from build123d import *

# Parameters (mm, degrees)
BOSS_EXTRUDE1_DEPTH = 50


with BuildPart() as part:
    # Sketch1 → Boss-Extrude1 (new body)
    with BuildSketch(Plane(origin=(0, 0, 0), x_dir=(1, 0, 0), z_dir=(0, 1, 0))):
        Polygon((-434.22123396, 330.511591748), (-490.415824699, -64.194072769), (-472.477870031, -524.138824529), (-270.660991621, -696.876695154), (273.24324441, -696.876695154), (475.06012282, -524.138824529), (492.998077488, -64.194072769), (436.803486749, 330.511591748), (255.52688097, 580.827312496), (1.291126394, 709.058947943), (-252.944628181, 580.827312496), align=None)
        Polygon((327.5, -536.876695154), (212.5, -536.876695154), (212.5, -411.876695154), (97.5, -411.876695154), (-97.5, -411.876695154), (-212.5, -411.876695154), (-212.5, -536.876695154), (-327.5, -536.876695154), (-327.5, -216.876695154), (-212.5, -216.876695154), (-212.5, -96.876695154), (-212.5, -81.876695154), (-317.5, -81.876695154), (-317.5, 118.123304846), (-202.5, 118.123304846), (-202.5, -81.876695154), (-202.5, -96.876695154), (-97.5, -96.876695154), (-97.5, -66.876695154), (97.5, -66.876695154), (97.5, -96.876695154), (202.5, -96.876695154), (202.5, -81.876695154), (202.5, 118.123304846), (317.5, 118.123304846), (317.5, -81.876695154), (212.5, -81.876695154), (212.5, -96.876695154), (212.5, -216.876695154), (327.5, -216.876695154), align=None, mode=Mode.SUBTRACT)
    extrude(amount=-BOSS_EXTRUDE1_DEPTH)


solid = part.part
Read the model definition and answer for the solid it produces. Units are mm, in the model's axes. A direction names the side the tool comes from. Round coordinates to 2 decimals unless told otherwise and drop trailing zeros. Order: outer loops, then holes, each group sorted by start corner. A loop starts at its lowest first (then second) coordinate and runs counter-clockwise, first axis right, second up.
1) For faces 1 (the face through (-261, -25, -118.123)), 2 (the face through (-124.05, -24.65, -645.84)), determine the directions among +Z, -Z, +X, -X, +Y, -Y from which every point of the face is accessible in a straight line to the end or side of a thin tool.
2) The part is cut by section D-D on z = -436.5. Write down the section's boundary in (x, y), plus the area to 3 significant figures.
3) Flat-ended cylindrical pins translate along their axes: pin 1 (15 mm diameter, centred on y = -25, z = 497, fed in from -X); pin 2 (8 mm diameter, centred on y = -27, z = -256.5, fed in from +X); pin 3 (24 mm diameter, centred on y = -22.5, z = 89.5, fed in from -X). Find the tip coordinate at first contact, or state that the pin passes through.
4) Straight lines are drawn through the part: L1, parallel to Z at x = -242.5, y = -26; L2, parallel to X at y = -31, z = 28.5; L3, parallel to Z at x = -262, y = -46. For each, find the intervals that lie inside material, in ascending order.
5) The part is cut by section B-B on z = 331. Write down the section's boundary in (x, y).
6) The mould has two halves that part along X. Classify faces 3 (the face through (-269, -25, 536.877)), 4 (the face through (-6, 0, -16)), 5 (the face through (327.5, -25, 375)), 6 (the face through (-461.925, -24.65, -135.922)): released by +X, released by -X, zero draft, split by the parting line, or undercut.
7) The part is cut by section A-A on x = -115. Write down the section's boundary in (y, z).
8) The part is cut by section C-C on z = -242.5. Write down the section's boundary in (x, y).
Resolved:
1. face 1: +Y, -Y
1. face 2: -Z, -X, +Y, -Y
2. outline: (-357.47, -50) - (360.05, -50) - (360.05, 0) - (-357.47, 0) - close
2. area: 35,900 mm2
3. pin 1: stops at x = -473.83
3. pin 2: stops at x = 447.91
3. pin 3: stops at x = -489.9
4. L1: z = -586.1 to -118.12, 81.88 to 216.88, 536.88 to 696.88
4. L2: x = -485.33 to -317.5, -202.5 to 202.5, 317.5 to 487.92
4. L3: z = -568.32 to -118.12, 81.88 to 216.88, 536.88 to 696.88
5. outline: (-480.01, -50) - (-327.5, -50) - (-327.5, 0) - (-480.01, 0) - close; (327.5, -50) - (482.59, -50) - (482.59, 0) - (327.5, 0) - close
6. face 3: undercut
6. face 4: zero draft
6. face 5: undercut
6. face 6: released by -X
7. outline: (-50, -650.4) - (0, -650.4) - (0, 96.88) - (-50, 96.88) - close; (-50, 411.88) - (0, 411.88) - (0, 696.88) - (-50, 696.88) - close
8. outline: (-446.75, -50) - (449.33, -50) - (449.33, 0) - (-446.75, 0) - close
